from build123d import *

# Parameters (mm, degrees)
BOSS_EXTRUDE1_DEPTH     = 5.953125
SKETCH3_W               = 47.23204247
SKETCH3_H               = 13.081
CUT_EXTRUDE1_DEPTH      = 924.398153884
BOSS_EXTRUDE3_DEPTH     = 11.90625
F_1_4_CLEARANCE_HOLE1_D = 6.7564
SKETCH13_W              = 23.41954247
SKETCH13_H              = 28.3464
CUT_EXTRUDE2_DEPTH      = 924.398153884
SKETCH14_R              = 3.429
CUT_EXTRUDE3_DEPTH      = 913.667776704
F_1_4_CLEARANCE_HOLE2_D = 6.7564
CUT_EXTRUDE4_DEPTH      = 913.667776704
BOSS_EXTRUDE4_START     = -11.90625
BOSS_EXTRUDE4_DEPTH     = 11.90625
BOSS_EXTRUDE5_DEPTH     = 11.90625
CUT_EXTRUDE5_DEPTH      = 912.387123535
FILLET1_R               = 3.3782


with BuildPart() as part:
    # Sketch1 → Boss-Extrude1 (new, symmetric)
    with BuildSketch(Plane.XY):
        Polygon((0, 0), (-396.875, 787.4), (-482.20704247, 787.4), (-85.33204247, 0), align=None)
    extrude(amount=BOSS_EXTRUDE1_DEPTH, both=True)

    # Sketch3 → Cut-Extrude1 (cut, through all)
    with BuildSketch(Plane.XY.offset(5.953125)):
        with Locations((-252.216021235, 371.4115)):
            Rectangle(SKETCH3_W, SKETCH3_H)
        with Locations((-444.303521235, 752.5131)):
            Rectangle(SKETCH3_W, SKETCH3_H)
    extrude(amount=-CUT_EXTRUDE1_DEPTH, mode=Mode.SUBTRACT)

    # Sketch10 → Boss-Extrude3 (add)
    with BuildSketch(Plane.XY.offset(5.953125)):
        with BuildLine():
            Line((-244.024703128, 501.780299783), (-249.740869802, 513.121174464))
            ThreePointArc((-249.740869802, 513.121174464), (-246.928515798, 521.649695143), (-238.39999512, 518.837341139))
            Line((-238.39999512, 518.837341139), (-226.967661771, 496.155591775))
            Line((-226.967661771, 496.155591775), (-239.680416455, 475.525946247))
            Line((-239.680416455, 475.525946247), (-251.112749804, 498.207695611))
            ThreePointArc((-251.112749804, 498.207695611), (-245.78242438, 496.449974359), (-244.024703128, 501.780299783))
        make_face()
        with BuildLine():
            Line((-351.145666605, 696.673002545), (-362.577999954, 719.354751908))
            ThreePointArc((-362.577999954, 719.354751908), (-357.24767453, 717.597030656), (-355.489953278, 722.92735608))
            Line((-355.489953278, 722.92735608), (-361.206119952, 734.268230762))
            ThreePointArc((-361.206119952, 734.268230762), (-358.393765948, 742.79675144), (-349.86524527, 739.984397436))
            Line((-349.86524527, 739.984397436), (-338.432911921, 717.302648072))
            Line((-338.432911921, 717.302648072), (-351.145666605, 696.673002545))
        make_face()
        with BuildLine():
            Line((0, 0), (-11.432333349, 22.681749364))
            ThreePointArc((-11.432333349, 22.681749364), (-6.102007925, 20.924028111), (-4.344286673, 26.254353535))
            Line((-4.344286673, 26.254353535), (-10.060453347, 37.595228217))
            ThreePointArc((-10.060453347, 37.595228217), (-7.248099343, 46.123748895), (1.280421335, 43.311394892))
            Line((1.280421335, 43.311394892), (12.712754684, 20.629645528))
            Line((12.712754684, 20.629645528), (23.110761502, 0))
            Line((23.110761502, 0), (0, 0))
        make_face()
    extrude(amount=-BOSS_EXTRUDE3_DEPTH)

    # 1/4 Clearance Hole1 (through all)
    with Locations(Plane.XY.offset(5.953125)):
        with Locations((-99.918593468, 162.967911886), (-427.0375, 720.5726), (-395.2875, 720.5726), (-203.2, 339.471), (-234.95, 339.471), (-69.85, 25.4), (-38.1, 25.4)):
            Hole(F_1_4_CLEARANCE_HOLE1_D / 2)

    # Sketch13 → Cut-Extrude2 (cut, through all)
    with BuildSketch(Plane.XY.offset(5.953125)):
        with Locations((-470.497271235, 773.2268)):
            Rectangle(SKETCH13_W, SKETCH13_H)
    extrude(amount=-CUT_EXTRUDE2_DEPTH, mode=Mode.SUBTRACT)

    # Sketch14 → Cut-Extrude3 (cut, through all)
    with BuildSketch(Plane.XY.offset(5.953125)):
        with Locations((-424.1165, 759.0536)):
            Circle(SKETCH14_R)
        with Locations((-424.1165, 745.9726)):
            Circle(SKETCH14_R)
        with Locations((-232.029, 377.952)):
            Circle(SKETCH14_R)
        with Locations((-232.029, 364.871)):
            Circle(SKETCH14_R)
    extrude(amount=-CUT_EXTRUDE3_DEPTH, mode=Mode.SUBTRACT)

    # 1/4 Clearance Hole2 (through all)
    with Locations(Plane.XY.offset(5.953125)):
        with Locations((-447.675, 736.6), (-449.2625, 774.7)):
            Hole(F_1_4_CLEARANCE_HOLE2_D / 2)

    # Sketch18 → Cut-Extrude4 (cut, through all)
    with BuildSketch(Plane.XY.offset(5.953125)):
        Polygon((-458.7875, 745.9726), (-458.7875, 740.93562774), (-461.326296502, 745.9726), align=None)
    extrude(amount=-CUT_EXTRUDE4_DEPTH, mode=Mode.SUBTRACT)

    # Sketch19 → Boss-Extrude4 (add)
    with BuildSketch(Plane(origin=(0, 0, -5.953125), x_dir=(-1, 0, 0), z_dir=(0, 0, -1)).offset(BOSS_EXTRUDE4_START)):
        with BuildLine():
            Line((458.7875, 759.0536), (458.7875, 745.9726))
            Line((458.7875, 745.9726), (427.5455, 745.9726))
            ThreePointArc((427.5455, 745.9726), (424.1165, 742.5436), (420.6875, 745.9726))
            Line((420.6875, 745.9726), (420.6875, 759.0536))
            ThreePointArc((420.6875, 759.0536), (424.1165, 762.4826), (427.5455, 759.0536))
            Line((427.5455, 759.0536), (458.7875, 759.0536))
        make_face()
        with BuildLine():
            Line((269.238796502, 364.871), (275.83204247, 377.952))
            Line((275.83204247, 377.952), (235.458, 377.952))
            ThreePointArc((235.458, 377.952), (232.029, 381.381), (228.6, 377.952))
            Line((228.6, 377.952), (228.6, 364.871))
            ThreePointArc((228.6, 364.871), (232.029, 361.442), (235.458, 364.871))
            Line((235.458, 364.871), (269.238796502, 364.871))
        make_face()
    extrude(amount=BOSS_EXTRUDE4_DEPTH)

    # Sketch20 → Boss-Extrude5 (add)
    with BuildSketch(Plane(origin=(0, 0, -5.953125), x_dir=(-1, 0, 0), z_dir=(0, 0, -1))):
        Polygon((349.86524527, 739.984397436), (361.206119952, 734.268230762), (364.064203289, 739.938668103), (352.723328607, 745.654834777), align=None)
        Polygon((238.39999512, 518.837341139), (249.740869802, 513.121174464), (252.598953139, 518.791611805), (241.258078457, 524.50777848), align=None)
        Polygon((-1.280421335, 43.311394892), (10.060453347, 37.595228217), (12.918536684, 43.265665558), (1.577662002, 48.981832233), align=None)
    extrude(amount=-BOSS_EXTRUDE5_DEPTH)

    # Sketch21 → Cut-Extrude5 (cut, through all)
    with BuildSketch(Plane(origin=(0, 0, -5.953125), x_dir=(-1, 0, 0), z_dir=(0, 0, -1))):
        Polygon((352.723328607, 745.654834777), (364.064203289, 739.938668103), (362.635161621, 737.103449432), (351.294286939, 742.819616107), align=None)
        Polygon((241.258078457, 524.50777848), (252.598953139, 518.791611805), (251.169911471, 515.956393135), (239.829036789, 521.672559809), align=None)
        Polygon((1.577662002, 48.981832233), (12.918536684, 43.265665558), (11.489495015, 40.430446888), (0.148620334, 46.146613562), align=None)
    extrude(amount=-CUT_EXTRUDE5_DEPTH, mode=Mode.SUBTRACT)

    # Fillet1
    fillet1_edges = [part.edges().sort_by_distance(p)[0] for p in [
        (-239.680416455, 475.525946247, 0),
        (-351.145666605, 696.673002545, 0),
    ]]
    fillet(fillet1_edges, radius=FILLET1_R)


solid = part.part
Work out the finished part from the listing and answer in its coordinate system (mm). Round coordinates to 2 decimals unless told otherwise and drop trailing zeros. Order: outer loops, then holes, each group sorted by start corner. A loop starts at its lowest first (then second) coordinate and runs counter-clockwise, first axis right, second up. Notation, with made-up numbers: M 53.25,45.5 L 76.25,45.5 A27 cw 76.25,67.5 Z; hole C 44,84 d5. An arc over 180 degrees is marked long. Put each result on its own line as item: value. Start each with the question number.
Q1. For a pull along X with two mould halves and no side action, classify faces 1 (the flat face through (-379.486, 752.901, 0.083)), 2 (the flat face through (-237, 396, -5.953)) as pulls with the +X half, pulls with the -X half, needs draft (parallel to the pull), parting line crosses it, or undercut.
Q2. Flat-ended cylindrical pins translate along their axes: pin 1 (5 mm diameter, centred on y = 223, z = 4, fed in from +X); pin 2 (6 mm diameter, centred on x = -29.5, z = 4.5, fed in from -Y); pin 3 (4 mm diameter, centred on y = 314.5, z = 2.5, fed in from -X); pin 4 (4 mm diameter, centred on x = -99.92, y = 162.97, fed in from +Z). Find the tip coordinate at first contact, or state that the pin passes through.
Q3. Straight lines are drawn through the part: L1, parallel to X at y = 738, z = -1.25; L2, parallel to X at y = 736.6, z = -1.75; L3, parallel to Y at x = -69.85, z = 0.25. For each, find the intervals that lie inside material, in ascending order. Write a range as [from, to].
Q4. Section C-C, the plane x = -380 is taken. Write down the section's boundary in (y, z).
Q5. Section B-B, the plane y = 205 is taken. Write down the section's boundary in (x, z), and give its area (3 significant figures).
Q6. Section A-A, the plane z = 1.25 is taken. Give the number of separate pieces and of enclosed holes in the cut face, and give its area (3 significant figures).
Findings below:
1. face 1: undercut
1. face 2: needs draft
2. pin 1: stops at x = -111.14
2. pin 2: stops at y = 0
2. pin 3: stops at x = -244.86
2. pin 4: passes through
3. L1: x = [-457.31, -450.75], [-444.6, -371.98], [-360.86, -348.87]
3. L2: x = [-456.6, -451.05], [-444.3, -371.27], [-362.38, -348.16]
3. L3: y = [0, 22.02], [28.78, 138.58]
4. outline: M 584.62,-5.95 L 753.92,-5.95 L 753.92,5.95 L 584.62,5.95 Z
5. outline: M -188.66,-5.95 L -103.33,-5.95 L -103.33,5.95 L -188.66,5.95 Z
5. area: 1,020 mm^2
6. separate pieces: 1
6. enclosed holes: 9
6. area: 68,300 mm^2
